CAD build for the part. Positions are in the model's coordinates, mm. Face numbers are marked on the shaded views. A direction names the side the tool comes from. Give positions to 0.01 mm unless a question says otherwise; leave off trailing zeros. Loops run counter-clockwise (first coordinate to the right, second up) from the corner with the lowest first, then second, coordinate; pieces in that order, holes last.
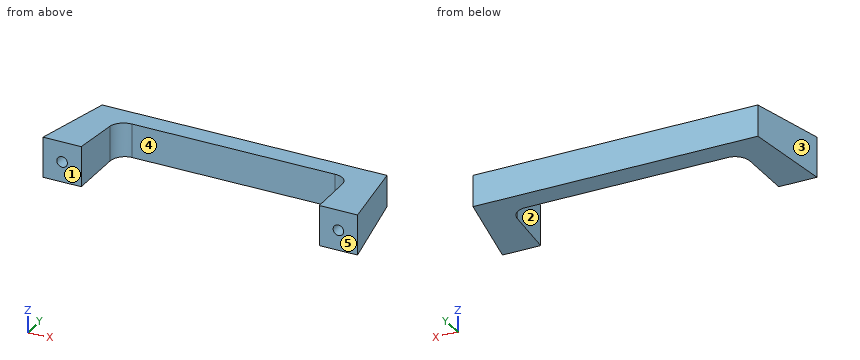
```python
from build123d import *

# Parameters (mm, degrees)
BOSS_EXTRUDE1_DEPTH = 19
DRAFT1_ANGLE        = 3


with BuildPart() as part:
    # Sketch1 → Boss-Extrude1 (new body)
    with BuildSketch(Plane.XY):
        with BuildLine():
            Line((-74, 0), (-67.013633203, 40))
            Line((-67.013633203, 40), (67.013633203, 40))
            Line((67.013633203, 40), (74, 0))
            Line((74, 0), (56, 0))
            Line((56, 0), (54.743185165, 23.37581641))
            ThreePointArc((54.743185165, 23.37581641), (52.568324233, 28.080881561), (47.753280872, 30))
            Line((47.753280872, 30), (-47.753280872, 30))
            ThreePointArc((-47.753280872, 30), (-52.568324233, 28.080881561), (-54.743185165, 23.37581641))
            Line((-54.743185165, 23.37581641), (-56, 0))
            Line((-56, 0), (-74, 0))
        make_face()
    extrude(amount=BOSS_EXTRUDE1_DEPTH)

    # Draft1
    draft1_faces = [part.faces().sort_by_distance(p)[0] for p in [
        (-68.996577663, 19.736222921, 0),
        (-68.996577663, 19.736222921, 19),
    ]]
    draft(draft1_faces, Plane.ZX, DRAFT1_ANGLE)

    # Sketch3 → M6x1.0 Tapped Hole1 (revolve, cut)
    with BuildSketch(Plane(origin=(-65, 0, 9.5), x_dir=(0, 0, -1), z_dir=(1, 0, 0))):
        Polygon((0, 0), (0, 16.502151548), (2.5, 15), (2.5, 0), align=None)
    m6x1_0_tapped_hole1 = revolve(axis=Axis((-65, -6.35, 9.5), (0, 1, 0)), mode=Mode.SUBTRACT)

    # Mirror1: M6x1.0 Tapped Hole1 across plane
    add(m6x1_0_tapped_hole1.mirror(Plane(origin=(0, 0, 0), x_dir=(0, 0, 1), z_dir=(1, 0, 0))), mode=Mode.SUBTRACT)


solid = part.part
```
1. Tool access for the marked faces 1 and 2: list every direction of +Z, -Z, +X, -X, +Y, -Y with a clear straight run to the whole face (end or side of a thin tool).
Responses:
face 1: +Z, -Z, +X, -X, -Y
face 2: +Z, -Z, -Y
2. Saw through at B-B, the plane y = 12. List the corners of the cut face in (x, z), and give its area (3 significant figures).
Responses:
outline: (-71.9, 0.63) - (-55.35, 0.63) - (-55.35, 18.37) - (-71.9, 18.37) - close; (55.35, 0.63) - (71.9, 0.63) - (71.9, 18.37) - (55.35, 18.37) - close; hole circle Ø5 at (-65, 9.5); hole circle Ø5 at (65, 9.5)
area: 548 mm2
3. Saw through at C-C, the plane x = 59.5. List the corners of the cut face in (y, z), and give its area (3 significant figures).
Responses:
outline: (0, 0) - (40, 2.1) - (40, 16.9) - (0, 19) - close
area: 676 mm2
4. Saw through at D-D, the plane x = 32. List the corners of the cut face in (y, z), and give its area (3 significant figures).
Responses:
outline: (30, 1.57) - (40, 2.1) - (40, 16.9) - (30, 17.43) - close
area: 153 mm2
5. Saw through at A-A, the plane z = 5.75. List the corners of the cut face in (x, y), and give its area (3 significant figures).
Responses:
outline: (-74, 0) - (-56, 0) - (-54.74, 23.38) arc R7 cw to (-47.75, 30) - (47.75, 30) arc R7 cw to (54.74, 23.38) - (56, 0) - (74, 0) - (67.01, 40) - (-67.01, 40) - close
area: 2,350 mm2
6. Probe line 1 along X through (y, z) = (7, 11.75); line 2 along X through (y, z) = (6.5, 9.5); line 3 along X through (y, z) = (20, 2.75). List the from-to ranges inside material, lowest first.
Responses:
line 1: x = -72.78 to -66.09, -63.91 to -55.62, 55.62 to 63.91, 66.09 to 72.78
line 2: x = -72.86 to -67.5, -62.5 to -55.65, 55.65 to 62.5, 67.5 to 72.86
line 3: x = -70.51 to -54.92, 54.92 to 70.51
7. Drop flat-ended pins along their axis: pin 1 (6 mm diameter, centred on x = 46, y = 29, fed in from -Z); pin 2 (2 mm diameter, centred on x = -58.5, y = 12.5, fed in from -Z); pin 3 (4 mm diameter, centred on x = 15, z = 11.5, fed in from -Y). Give the stop position or say it passes through.
Responses:
pin 1: stops at z = 1.57
pin 2: stops at z = 0.6
pin 3: stops at y = 30
8. Pull direction X, two halves, no side cores. Call the marked faces 3, 4 and 5: released by +X, released by -X, zero draft, split by the parting line, or undercut.
Responses:
face 3: released by -X
face 4: undercut
face 5: zero draft
